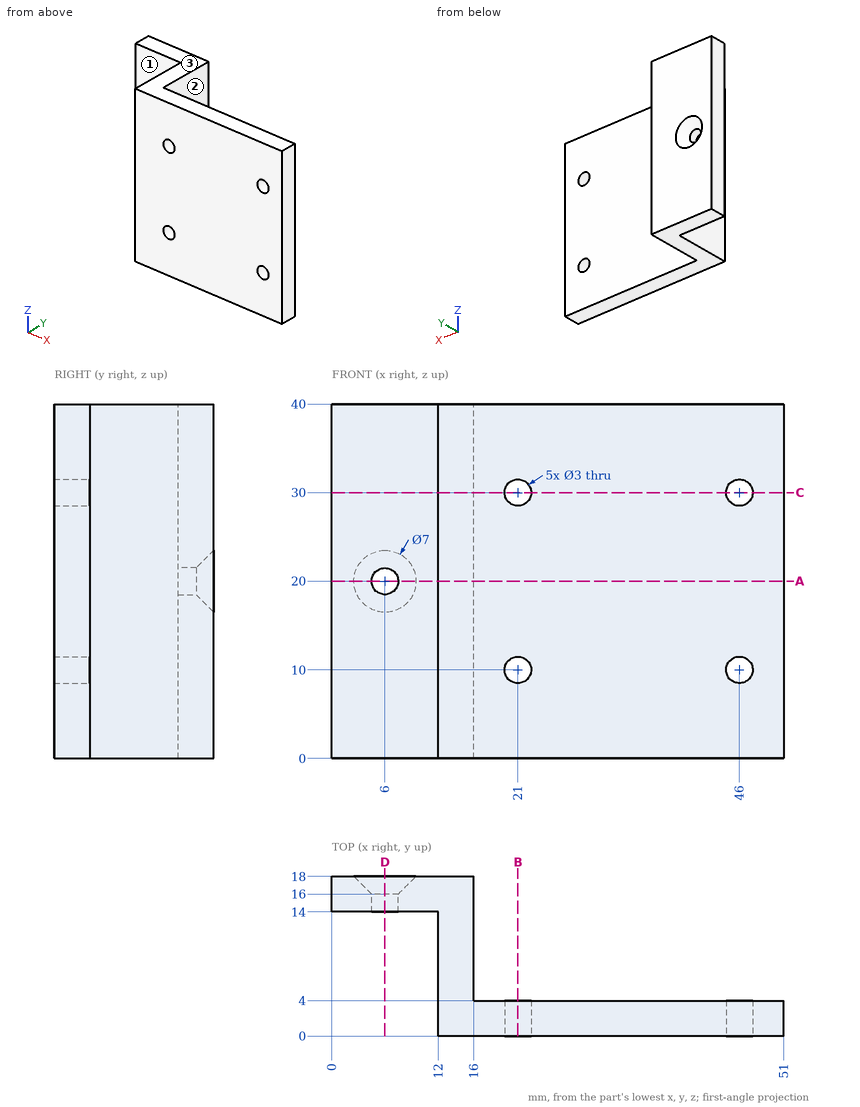
Check sheet for the drawn part. Datum: minimum x, y, z corner. Units: mm. A direction names the side the tool comes from. Round coordinates to 2 decimals unless told otherwise and drop trailing zeros. Order: outer loops, then holes, each group sorted by start corner. A loop starts at its lowest first (then second) coordinate and runs counter-clockwise, first axis right, second up.
1. Go/stop test with flat-tipped pins: P1, Ø4, axis at x = 37, z = 15, coming from the +Y side; P2, Ø10, axis at y = 5, z = 27, coming from the -X side; P3, Ø4, axis at y = 13, z = 17, coming from the +X side; P4, Ø2.5, axis at x = 46, z = 10, coming from the -Y side. Record where each tip stops, or that it passes through.
Final values:
P1: stops at y = 4
P2: stops at x = 12
P3: stops at x = 16
P4: passes through
2. Section check C-C on z = 30. Record the cut outline in (x, y), then the cut area to 3 significant figures.
Final values:
outline: (0, 14) - (12, 14) - (12, 0) - (19.5, 0) - (19.5, 4) - (16, 4) - (16, 18) - (0, 18) - close; (22.5, 0) - (44.5, 0) - (44.5, 4) - (22.5, 4) - close; (47.5, 0) - (51, 0) - (51, 4) - (47.5, 4) - close
area: 236 mm2
3. Section check A-A on z = 20. Record the cut outline in (x, y), then the cut area to 3 significant figures.
Final values:
outline: (0, 14) - (4.5, 14) - (4.5, 16) - (2.5, 18) - (0, 18) - close; (7.5, 14) - (12, 14) - (12, 0) - (51, 0) - (51, 4) - (16, 4) - (16, 18) - (9.5, 18) - (7.5, 16) - close
area: 244 mm2
4. Section check D-D on x = 6. Record the cut outline in (y, z).
Final values:
outline: (14, 0) - (18, 0) - (18, 16.5) - (16, 18.5) - (14, 18.5) - close; (14, 21.5) - (16, 21.5) - (18, 23.5) - (18, 40) - (14, 40) - close
5. Thickness scan on L1, parallel to X at y = 3.25, z = 30; L2, parallel to X at y = 15.15, z = 20; L3, parallel to X at y = 6.75, z = 31. Record the ranges inside material, lowest first.
Final values:
L1: x = 12 to 19.5, 22.5 to 44.5, 47.5 to 51
L2: x = 0 to 4.5, 7.5 to 16
L3: x = 12 to 16
6. Access from +Z, -Z, +X, -X, +Y, -Y to the whole of each face (thin tool, end or side, straight path). Record for the marked faces 1, 2 and 3.
Final values:
face 1: +Z, -Z, -X, -Y
face 2: +Z, -Z, +X, +Y
face 3: +Z, +X, -X, +Y, -Y
7. Section check B-B on x = 21. Record the cut outline in (y, z).
Final values:
outline: (0, 0) - (4, 0) - (4, 8.5) - (0, 8.5) - close; (0, 11.5) - (4, 11.5) - (4, 28.5) - (0, 28.5) - close; (0, 31.5) - (4, 31.5) - (4, 40) - (0, 40) - close
